Here's how the part is built. I have some questions about the finished solid (model axes, mm). Face numbers are marked on the shaded views. A direction names the side the tool comes from. Round coordinates to 2 decimals unless told otherwise and drop trailing zeros. Order: outer loops, then holes, each group sorted by start corner. A loop starts at its lowest first (then second) coordinate and runs counter-clockwise, first axis right, second up. Notation, with made-up numbers: (-25.75, 53.5) - (-11.75, 53.5) arc R30 cw to (-11.75, 81.5) - close; hole circle Ø2 at (-32, 1). An arc over 180 degrees is marked (long way). One line per item, written item: value.
from build123d import *

# Parameters (mm, degrees)
SKETCH1_R                = 16.5
SKETCH1_R_2              = 8.5
BOSS_EXTRUDE1_DEPTH      = 15.5
SKETCH2_R                = 16.5
SKETCH2_R_2              = 2.15
BOSS_EXTRUDE2_DEPTH      = 3
BOSS_EXTRUDE2_DEPTH_BACK = 1
CHAMFER2_SIZE            = 0.5
CHAMFER3_SIZE            = 2


with BuildPart() as part:
    # Sketch1 → Boss-Extrude1 (new body)
    with BuildSketch(Plane(origin=(0, 0, 0), x_dir=(1, 0, 0), z_dir=(0, 1, 0))):
        Circle(SKETCH1_R)
        Circle(SKETCH1_R_2, mode=Mode.SUBTRACT)
    extrude(amount=BOSS_EXTRUDE1_DEPTH)

    # Sketch2 → Boss-Extrude2 (add, two sides)
    with BuildSketch(Plane.XZ) as boss_extrude2_sk:
        Circle(SKETCH2_R)
        Circle(SKETCH2_R_2, mode=Mode.SUBTRACT)
    extrude(amount=BOSS_EXTRUDE2_DEPTH)
    extrude(boss_extrude2_sk.sketch, amount=-BOSS_EXTRUDE2_DEPTH_BACK)

    # Chamfer2
    chamfer2_edges = [part.edges().sort_by_distance(p)[0] for p in [
        (-16.5, -3, 0),
        (-16.5, 15.5, 0),
        (-8.5, 15.5, 0),
    ]]
    chamfer(chamfer2_edges, length=CHAMFER2_SIZE)

    # Chamfer3
    chamfer3_edges = [part.edges().sort_by_distance(p)[0] for p in [
        (-8.5, 1, 0),
    ]]
    chamfer(chamfer3_edges, length=CHAMFER3_SIZE)


solid = part.part
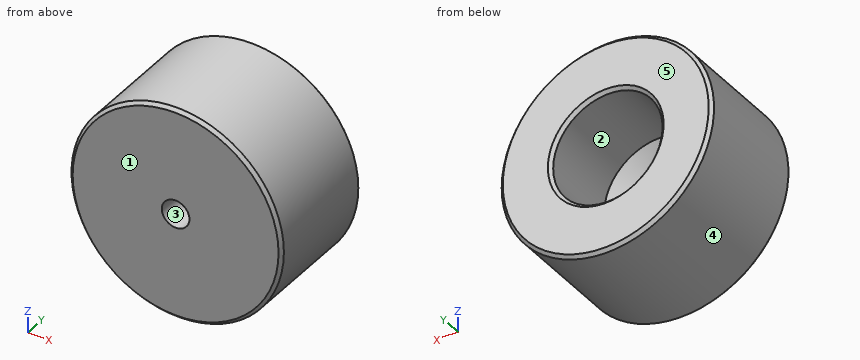
Q1. If we section it at D-D, the plane y = 0: Please give me the cut outline in (x, z), then the cut area to 3 significant figures.
Results list:
outline: circle Ø33 at (0, 0); hole circle Ø4.3 at (0, 0)
area: 841 mm²
Q2. We'd pull the mould along Z, two halves only. Please class the marked faces 3, 4 and 5: released by +Z, released by -Z, zero draft, split by the parting line, or undercut.
Results list:
face 3: undercut
face 4: split by the parting line
face 5: zero draft
Q3. Will these pins go through, and if not, where does the flat tip stop? pin 1 (1.5 mm diameter, centred on y = 9, z = -10.5, fed in from -X); pin 2 (1.5 mm diameter, centred on y = 3.5, z = 13, fed in from -X); pin 3 (4 mm diameter, centred on x = -1, z = -2.5, fed in from +Y).
Results list:
pin 1: x = -13.31
pin 2: x = -11.05
pin 3: y = 1
Q4. Which directions (+Z, -Z, +X, -X, +Y, -Y) give clear straight access to the entire face, cutting with the end or side of a thin tool? Please do the marked faces 1 and 2.
Results list:
face 1: +Z, -Z, +X, -X, -Y
face 2: +Y
Q5. If we section it at A-A, the plane x = 0: Please give me the cut outline in (y, z), then the cut area to 3 significant figures.
Results list:
outline: (-3, -16) - (-2.5, -16.5) - (15, -16.5) - (15.5, -16) - (15.5, -9) - (15, -8.5) - (3, -8.5) - (1, -6.5) - (1, -2.15) - (-3, -2.15) - close; (-3, 2.15) - (1, 2.15) - (1, 6.5) - (3, 8.5) - (15, 8.5) - (15.5, 9) - (15.5, 16) - (15, 16.5) - (-2.5, 16.5) - (-3, 16) - close
area: 350 mm²
Q6. If I drill on line 1 along Z through (x, y) = (0, 11.75); line 2 along Z through (x, y) = (0, -2), over which ranges is the centre line in solid material (lowest first)?
Results list:
line 1: -16.5 to -8.5, 8.5 to 16.5
line 2: -16.5 to -2.15, 2.15 to 16.5
Q7. If we section it at C-C, the plane y = 4: Please give me the cut outline in (x, z).
Results list:
outline: circle Ø33 at (0, 0); hole circle Ø17 at (0, 0)
Q8. If we section it at B-B, the plane z = 0: Please give me the cut outline in (x, y).
Results list:
outline: (-16.5, -2.5) - (-16, -3) - (-2.15, -3) - (-2.15, 1) - (-6.5, 1) - (-8.5, 3) - (-8.5, 15) - (-9, 15.5) - (-16, 15.5) - (-16.5, 15) - close; (2.15, -3) - (16, -3) - (16.5, -2.5) - (16.5, 15) - (16, 15.5) - (9, 15.5) - (8.5, 15) - (8.5, 3) - (6.5, 1) - (2.15, 1) - close
